Could you check a few things on this model? Use its own coordinates, in mm. A direction names the side the tool comes from. Give positions to 0.01 mm unless a question says otherwise; leave off trailing zeros. Write each loop counter-clockwise with the first axis right and the second up, starting at its lowest first coordinate (ties: lowest second). Pieces come first, ordered by that corner, then holes. Notation, with made-up numbers: M -27,-9.5 L -4,-9.5 A14 ccw -4,4.5 Z; hole C 19,2 d10. An arc over 180 degrees is marked long. Write each question's results on one line, items separated by ' | '. Start each with the question number.
from build123d import *

# Parameters (mm, degrees)
EXTRUDE_1_DEPTH     = 12
SKETCH_3_R          = 11
CUT_EXTRUDE_1_DEPTH = 179.941331168
CUT_EXTRUDE_START   = -5
CUT_EXTRUDE_2_DEPTH = 5
CUT_EXTRUDE_START_2 = -4
CUT_EXTRUDE_3_DEPTH = 4
SKETCH_6_R          = 2.5
CUT_EXTRUDE_4_DEPTH = 160.561900214
FILLET_1_R          = 3
FILLET_2_R          = 3
SKETCH_7_R          = 1.5
CUT_EXTRUDE_6_DEPTH = 179.941331168


with BuildPart() as part:
    # 草图1 → 拉伸1 (new body)
    with BuildSketch(Plane.XY):
        with BuildLine():
            Line((0, -40), (0, -26))
            ThreePointArc((0, -26), (26, 0), (0, 26))
            Line((0, 26), (0, 40))
            Line((0, 40), (20, 40))
            Line((20, 40), (20, 28))
            Line((20, 28), (149.800932204, 10.911383086))
            ThreePointArc((149.800932204, 10.911383086), (150.911506836, 10.973150989), (151.923244173, 11.435296905))
            ThreePointArc((151.923244173, 11.435296905), (174, 0), (151.923244173, -11.435296905))
            ThreePointArc((151.923244173, -11.435296905), (150.911506836, -10.973150989), (149.800932204, -10.911383086))
            Line((149.800932204, -10.911383086), (20, -28))
            Line((20, -28), (20, -40))
            Line((20, -40), (0, -40))
        make_face()
    extrude(amount=EXTRUDE_1_DEPTH)

    # 草图3 → 切除-拉伸1 (cut, through all)
    with BuildSketch(Plane.XY.offset(12)):
        with Locations((160, 0)):
            Circle(SKETCH_3_R)
    extrude(amount=-CUT_EXTRUDE_1_DEPTH, mode=Mode.SUBTRACT)

    # 草图4 → 切除-拉伸2 (cut)
    with BuildSketch(Plane.XY.offset(12).offset(CUT_EXTRUDE_START)):
        with BuildLine():
            Line((0, 40), (0, 31))
            ThreePointArc((0, 31), (31, 0), (0, -31))
            Line((0, -31), (0, -40))
            Line((0, -40), (20, -40))
            Line((20, -40), (20, -28))
            Line((20, -28), (149.800932204, -10.911383086))
            ThreePointArc((149.800932204, -10.911383086), (150.911506836, -10.973150989), (151.923244173, -11.435296905))
            ThreePointArc((151.923244173, -11.435296905), (146, 0), (151.923244173, 11.435296905))
            ThreePointArc((151.923244173, 11.435296905), (150.911506836, 10.973150989), (149.800932204, 10.911383086))
            Line((149.800932204, 10.911383086), (20, 28))
            Line((20, 28), (20, 40))
            Line((20, 40), (0, 40))
        make_face()
    extrude(amount=CUT_EXTRUDE_2_DEPTH, mode=Mode.SUBTRACT)

    # 草图5 → 切除-拉伸3 (cut)
    with BuildSketch(Plane.XY.offset(7).offset(CUT_EXTRUDE_START_2)):
        with BuildLine():
            Line((143.607465988, 5.674994619), (29.398745634, 20.7108579))
            ThreePointArc((29.398745634, 20.7108579), (26.491956539, 19.371673477), (26.44771114, 16.171535964))
            ThreePointArc((26.44771114, 16.171535964), (31, 0), (26.44771114, -16.171535964))
            ThreePointArc((26.44771114, -16.171535964), (26.491956539, -19.371673477), (29.398745634, -20.7108579))
            Line((29.398745634, -20.7108579), (143.607465988, -5.674994619))
            ThreePointArc((143.607465988, -5.674994619), (145.621853626, -4.492677495), (146.177789633, -2.22407297))
            ThreePointArc((146.177789633, -2.22407297), (146, 0), (146.177789633, 2.22407297))
            ThreePointArc((146.177789633, 2.22407297), (145.621853626, 4.492677495), (143.607465988, 5.674994619))
        make_face()
    extrude(amount=CUT_EXTRUDE_3_DEPTH, mode=Mode.SUBTRACT)

    # 镜向1: part across plane


with BuildPart() as part_1:
    add(part.part)
    add(part.part.mirror(Plane.XY))

    # 草图6 → 切除-拉伸4 (cut, through all)
    with BuildSketch(Plane(origin=(20, 0, 0), x_dir=(0, 0, -1), z_dir=(1, 0, 0))):
        with Locations((0, -34)):
            Circle(SKETCH_6_R)
    cut_extrude_4 = extrude(amount=-CUT_EXTRUDE_4_DEPTH, mode=Mode.SUBTRACT)

    # 镜向2: 切除-拉伸4 across plane
    add(cut_extrude_4.mirror(Plane.ZX), mode=Mode.SUBTRACT)

    # 圆角1
    fillet_1_edges = [part_1.edges().sort_by_distance(p)[0] for p in [
        (10, 40, 7),
        (10, -40, 7),
        (31, 0, 12),
        (26.491956539, 19.371673477, 3),
        (86.503105811, 13.192926259, 3),
        (145.621853626, 4.492677495, 3),
        (146, 0, 3),
        (145.621853626, -4.492677495, 3),
        (86.503105811, -13.192926259, 3),
        (26.491956539, -19.371673477, 3),
        (31, 0, 3),
    ]]
    fillet(fillet_1_edges, radius=FILLET_1_R)

    # 圆角2
    fillet_2_edges = [part_1.edges().sort_by_distance(p)[0] for p in [
        (10, 40, -7),
        (10, -40, -7),
        (146, 0, -3),
        (31, 0, -12),
        (31, 0, -3),
        (26.491956539, 19.371673477, -3),
        (86.503105811, 13.192926259, -3),
        (145.621853626, 4.492677495, -3),
        (145.621853626, -4.492677495, -3),
        (86.503105811, -13.192926259, -3),
        (26.491956539, -19.371673477, -3),
    ]]
    fillet(fillet_2_edges, radius=FILLET_2_R)

    # 草图7 → 切除-拉伸6 (cut, through all)
    with BuildSketch(Plane(origin=(0, 0, 0), x_dir=(0, 0, -1), z_dir=(1, 0, 0))):
        with Locations(Location((0, 0, 0), (0, 0, 180))):
            Circle(SKETCH_7_R)
    extrude(amount=CUT_EXTRUDE_6_DEPTH, mode=Mode.SUBTRACT)


solid = part_1.part
Q1. For faces 1 (the face through (70, 20, 7)), 2 (the face through (85.7, -13.3, -6.5)), 3 (the face through (20, -31, 0)), 4 (the face through (87.19, -12.24, 3.9)), which set-ups out of +Z, -Z, +X, -X, +Y, -Y let a thin tool reach every point of the face, with its end or its side?
Q2. If we mould it in two halves opening along X, with no side actions, what happens to faces 5 (the face through (26.467, -19.332, 6.493)), 6 (the face through (153.8, -9.3, 12)), 7 (the face through (0, 31, 0)), 8 (the face through (87.3, 13.09, -6.49))? For each: pulls with the +X half, pulls with the -X half, needs draft (parallel to the pull), parting line crosses it, or undercut.
Q3. I'm going to push flat-ended pins straight in: P1, Ø1.5, axis at y = 0, z = -4, coming from the -X side; P2, Ø10, axis at x = 134.5, z = -6, coming from the +Y side; P3, Ø10.5, axis at x = 74.5, y = -14.5, coming from the -Z side; P4, Ø4, axis at y = -34, z = 0, coming from the +X side. Where does each tip first touch, or does it pass through?
Q4. Please list where these lines run through material, in increasing order: line 1 (Y direction, x = 160, z = -6.25); line 2 (X direction, y = -3, z = 5.25); line 3 (Y direction, x = 9.75, z = 0). Write a range as [from, to].
Q5. If we section it at A-A (x = 160): Please give me the cut outline in (y, z).
Determined:
1) face 1: +Z, +Y | face 2: -Z | face 3: +Z, -Z, +X, -Y | face 4: +Z
2) face 5: undercut | face 6: needs draft | face 7: pulls with the -X half | face 8: undercut
3) P1: stops at x = 25.99 | P2: stops at y = 13.58 | P3: stops at z = -7 | P4: passes through
4) line 1: y = [-14, -11], [11, 14] | line 2: x = [25.83, 30.95], [146.11, 149.42], [170.58, 173.67] | line 3: y = [-40, -36.5], [-31.5, -24.1], [24.1, 31.5], [36.5, 40]
5) outline: M -14,-12 L -11,-12 L -11,12 L -14,12 Z; M 11,-12 L 14,-12 L 14,12 L 11,12 Z
